from build123d import *

# Parameters (mm, degrees)
SKETCH2_R           = 4
SKETCH2_R_2         = 1.5
BOSS_EXTRUDE1_DEPTH = 3
SKETCH3_W           = 26
SKETCH3_H           = 3
BOSS_EXTRUDE2_DEPTH = 31
SKETCH4_R           = 5
SKETCH4_R_2         = 1.5
CUT_EXTRUDE1_DEPTH  = 48.16990566
FILLET1_R           = 3
FILLET2_R           = 3


with BuildPart() as part:
    # Sketch2 → Boss-Extrude1 (new body)
    with BuildSketch(Plane.XY):
        with BuildLine():
            Line((-13, 0), (13, 0))
            Line((13, 0), (13, 20))
            ThreePointArc((13, 20), (0, 33), (-13, 20))
            Line((-13, 20), (-13, 0))
        make_face()
        with Locations((0, 20)):
            Circle(SKETCH2_R, mode=Mode.SUBTRACT)
        with Locations((-8.5, 20)):
            Circle(SKETCH2_R_2, mode=Mode.SUBTRACT)
        with Locations((8.5, 20)):
            Circle(SKETCH2_R_2, mode=Mode.SUBTRACT)
    extrude(amount=BOSS_EXTRUDE1_DEPTH)

    # Sketch3 → Boss-Extrude2 (add)
    with BuildSketch(Plane.XY.offset(3)):
        with Locations((0, 1.5)):
            Rectangle(SKETCH3_W, SKETCH3_H)
    extrude(amount=BOSS_EXTRUDE2_DEPTH)

    # Sketch4 → Cut-Extrude1 (cut, through all)
    with BuildSketch(Plane(origin=(0, 3, 0), x_dir=(1, 0, 0), z_dir=(0, 1, 0))):
        with Locations(Location((0, -18.5, 0), (0, 0, 180))):
            Circle(SKETCH4_R)
        with Locations(Location((-8, -11.5, 0), (0, 0, 180))):
            Circle(SKETCH4_R_2)
        with Locations(Location((8, -11.5, 0), (0, 0, 180))):
            Circle(SKETCH4_R_2)
        with Locations(Location((8, -25.5, 0), (0, 0, 180))):
            Circle(SKETCH4_R_2)
        with Locations(Location((-8, -25.5, 0), (0, 0, 180))):
            Circle(SKETCH4_R_2)
    extrude(amount=-CUT_EXTRUDE1_DEPTH, mode=Mode.SUBTRACT)

    # Fillet1
    fillet1_edges = [part.edges().sort_by_distance(p)[0] for p in [
        (-13, 1.5, 34),
        (13, 1.5, 34),
    ]]
    fillet(fillet1_edges, radius=FILLET1_R)

    # Fillet2
    fillet2_edges = [part.edges().sort_by_distance(p)[0] for p in [
        (0, 0, 0),
    ]]
    fillet(fillet2_edges, radius=FILLET2_R)


solid = part.part
Source: CAD feature listing. Evaluate the final solid. Frame: model axes, mm. A direction names the side the tool comes from. Round coordinates to 2 decimals unless told otherwise and drop trailing zeros. Loops run counter-clockwise (first coordinate to the right, second up) from the corner with the lowest first, then second, coordinate; pieces in that order, holes last. Notation, with made-up numbers: (65.25, 74.25) -> (111.25, 74.25) arc R16 ccw to (111.25, 103.25) -> close; hole circle Ø2 at (49, 40.25). An arc over 180 degrees is marked (long way). Answer as a JSON object with one key per item and string values. Group by question number.
Q1. Contact query for flat-ended pins moving along their axis: P1, Ø8, axis at x = -1, z = 16, coming from the +Y side; P2, Ø13, axis at x = 2, y = 21.5, coming from the +Z side. Output: stop coordinate, or through.
Q2. Section query D-D (x = -8). Output: boundary loops of the cut face in (y, z), plus the area to 3 significant figures.
Q3. Section query B-B (z = 18.5). Output: boundary loops of the cut face in (x, y), plus the area to 3 significant figures.
Q4. Ray query, line 1 (Z direction, x = -8, y = 2.25); line 2 (X direction, y = 2.5, z = 24.5); line 3 (X direction, y = 1, z = 11). Return the intervals inside material, ascending. Write a range as from..to.
Q5. Mould query, pull axis Y, two halves, no side actions, for faces 3 (the cylindrical face through (0.18, 0.86, 0.9)), 4 (the cylindrical face through (-0.521, 23.966, 1.479)), 5 (the cylindrical face through (8, 2, 27)). Classes: pulls with the +Y half, pulls with the -Y half, needs draft (parallel to the pull), parting line crosses it, or undercut.
Q6. Section query A-A (x = 0). Output: boundary loops of the cut face in (y, z).
Q7. Access query for faces 1 (the cylindrical face through (-12.14, 1.52, 33.1)), 2 (the flat face through (0, 15, 3)). Directions: +Z, -Z, +X, -X, +Y, -Y. A direction counts if a zero-diameter tool reaches every point of the face in a straight line with its end or side. Return the directions, or none.
Q8. Section query C-C (z = 24.5). Output: boundary loops of the cut face in (x, y).
Completed:
{
 "1": {"P1": "y = 3", "P2": "z = 3"},
 "2": {"outline": "(0, 3) arc R3 ccw to (3, 0) -> (18.59, 0) -> (18.59, 3) -> (3, 3) -> (3, 10) -> (0, 10) -> close; (0, 13) -> (3, 13) -> (3, 24) -> (0, 24) -> close; (0, 27) -> (3, 27) -> (3, 34) -> (0, 34) -> close; (21.41, 0) -> (30.25, 0) -> (30.25, 3) -> (21.41, 3) -> close", "area": "155 mm²"},
 "3": {"outline": "(-13, 0) -> (-5, 0) -> (-5, 3) -> (-13, 3) -> close; (5, 0) -> (13, 0) -> (13, 3) -> (5, 3) -> close", "area": "48.0 mm²"},
 "4": {"line 1": "0.1..10, 13..24, 27..34", "line 2": "-13..-9.12, -6.88..6.88, 9.12..13", "line 3": "-13..-9.41, -6.59..6.59, 9.41..13"},
 "5": {"face 3": "pulls with the -Y half", "face 4": "undercut", "face 5": "needs draft"},
 "6": {"outline": "(0, 3) arc R3 ccw to (3, 0) -> (16, 0) -> (16, 3) -> (3, 3) -> (3, 13.5) -> (0, 13.5) -> close; (0, 23.5) -> (3, 23.5) -> (3, 34) -> (0, 34) -> close; (24, 0) -> (33, 0) -> (33, 3) -> (24, 3) -> close"},
 "7": {"face 1": "+Z, -X, +Y, -Y", "face 2": "+Z, +X, -X, +Y"},
 "8": {"outline": "(-13, 0) -> (-9.12, 0) -> (-9.12, 3) -> (-13, 3) -> close; (-6.88, 0) -> (6.88, 0) -> (6.88, 3) -> (-6.88, 3) -> close; (9.12, 0) -> (13, 0) -> (13, 3) -> (9.12, 3) -> close"}
}
